```python
from build123d import *

# Parameters (mm, degrees)
SKETCH3_R           = 90
BOSS_EXTRUDE3_DEPTH = 2
SKETCH4_R           = 45
CUT_EXTRUDE1_DEPTH  = 2
BOSS_EXTRUDE4_DEPTH = 85
BOSS_EXTRUDE5_DEPTH = 85
CUT_EXTRUDE9_DEPTH  = 10
CIRPATTERN4_COUNT   = 3
CUT_EXTRUDE5_DEPTH  = 60
SKETCH15_W          = 5
SKETCH15_H          = 25
CUT_EXTRUDE10_DEPTH = 88.0000001
CIRPATTERN5_COUNT   = 3
SKETCH16_R          = 46
CUT_EXTRUDE11_DEPTH = 85
BOSS_EXTRUDE6_DEPTH = 2
SKETCH18_W          = 18.5
SKETCH18_H          = 12
CUT_EXTRUDE12_DEPTH = 2


with BuildPart() as part:
    # Sketch3 → Boss-Extrude3 (new body)
    with BuildSketch(Plane(origin=(0, 0, 0), x_dir=(1, 0, 0), z_dir=(0, 1, 0))):
        Circle(SKETCH3_R)
    extrude(amount=BOSS_EXTRUDE3_DEPTH)

    # Sketch4 → Cut-Extrude1 (cut)
    with BuildSketch(Plane.XZ):
        Circle(SKETCH4_R)
    extrude(amount=-CUT_EXTRUDE1_DEPTH, mode=Mode.SUBTRACT)

    # Sketch6 → Boss-Extrude4 (add)
    with BuildSketch(Plane.XZ):
        with BuildLine():
            Line((-46, 0), (-45, 0))
            ThreePointArc((-45, 0), (-41.574578963, 17.220754456), (-31.819805153, 31.819805153))
            Line((-31.819805153, 31.819805153), (-32.526911935, 32.526911935))
            ThreePointArc((-32.526911935, 32.526911935), (-42.498458496, 17.603437889), (-46, 0))
        make_face()
    boss_extrude4 = extrude(amount=BOSS_EXTRUDE4_DEPTH)

    # Sketch6<3> → Boss-Extrude5 (add)
    with BuildSketch(Plane.XZ):
        with BuildLine():
            Line((-50, 0), (-48, 0))
            ThreePointArc((-48, 0), (-44.346217561, 18.368804754), (-33.941125497, 33.941125497))
            Line((-33.941125497, 33.941125497), (-35.355339059, 35.355339059))
            ThreePointArc((-35.355339059, 35.355339059), (-46.193976626, 19.134171618), (-50, 0))
        make_face()
    boss_extrude5 = extrude(amount=BOSS_EXTRUDE5_DEPTH)

    # Sketch14 → Cut-Extrude9 (cut)
    with BuildSketch(Plane(origin=(-38.409902577, 0, 15.909902577), x_dir=(-0.382683432, 0, -0.923879533), z_dir=(0.923879533, 0, -0.382683432))):
        with BuildLine():
            Line((1.5, -75), (1.5, -83))
            ThreePointArc((1.5, -83), (0, -84.5), (-1.5, -83))
            Line((-1.5, -83), (-1.5, -75))
            ThreePointArc((-1.5, -75), (0, -73.5), (1.5, -75))
        make_face()
    cut_extrude9 = extrude(amount=-CUT_EXTRUDE9_DEPTH, mode=Mode.SUBTRACT)

    # CirPattern4: Boss-Extrude4, Boss-Extrude5, Cut-Extrude9 ×3 about axis
    cirpattern4_axis = Axis((0, 0, 0), (0, 1, 0))
    for i in range(1, CIRPATTERN4_COUNT):
        add(boss_extrude4.rotate(cirpattern4_axis, i * 360 / CIRPATTERN4_COUNT))
        add(boss_extrude5.rotate(cirpattern4_axis, i * 360 / CIRPATTERN4_COUNT))
        add(cut_extrude9.rotate(cirpattern4_axis, i * 360 / CIRPATTERN4_COUNT), mode=Mode.SUBTRACT)

    # Sketch11 → Cut-Extrude5 (cut, symmetric)
    with BuildSketch(Plane.XZ):
        Polygon((-6.747570404, -52.479477871), (11.40662685, -48.919264104), (13.715954699, -60.69495962), (-4.438242555, -64.255173387), align=None)
    extrude(amount=CUT_EXTRUDE5_DEPTH, both=True, mode=Mode.SUBTRACT)

    # Sketch15 → Cut-Extrude10 (cut, through all)
    with BuildSketch(Plane(origin=(0, 2, 0), x_dir=(1, 0, 0), z_dir=(0, 1, 0))):
        with Locations((57.5, -4.067185812)):
            Rectangle(SKETCH15_W, SKETCH15_H)
    cut_extrude10 = extrude(amount=-CUT_EXTRUDE10_DEPTH, mode=Mode.SUBTRACT)

    # CirPattern5: Cut-Extrude10 ×3 about axis
    cirpattern5_axis = Axis((0, 0, 0), (0, 1, 0))
    for i in range(1, CIRPATTERN5_COUNT):
        add(cut_extrude10.rotate(cirpattern5_axis, i * 360 / CIRPATTERN5_COUNT), mode=Mode.SUBTRACT)

    # Sketch16 → Cut-Extrude11 (cut)
    with BuildSketch(Plane.XZ.offset(85)):
        Circle(SKETCH16_R)
    extrude(amount=-CUT_EXTRUDE11_DEPTH, mode=Mode.SUBTRACT)

    # Sketch17 → Boss-Extrude6 (add)
    with BuildSketch(Plane(origin=(0, 2, 0), x_dir=(1, 0, 0), z_dir=(0, 1, 0))):
        Polygon((13.715954699, 60.69495962), (-4.438242555, 64.255173387), (-6.747570404, 52.479477871), (11.40662685, 48.919264104), align=None)
    extrude(amount=-BOSS_EXTRUDE6_DEPTH)

    # Sketch18 → Cut-Extrude12 (cut)
    with BuildSketch(Plane(origin=(0, 2, 0), x_dir=(1, 0, 0), z_dir=(0, 1, 0))):
        with Locations((9.25, -56)):
            Rectangle(SKETCH18_W, SKETCH18_H)
    extrude(amount=-CUT_EXTRUDE12_DEPTH, mode=Mode.SUBTRACT)


solid = part.part
```
The model under review builds one solid part; all positions refer to its coordinate system, in mm. A direction names the side the tool comes from. Coordinates: 2 decimals unless noted, no trailing zeros. Write each loop counter-clockwise with the first axis right and the second up, starting at its lowest first coordinate (ties: lowest second). Pieces come first, ordered by that corner, then holes.
1) We need section A-A on y = -6. State the section outline as (x, z) points.
2) We need section C-C on x = -2.5. State the section outline as (y, z) points, then the cut area to 3 significant figures.
3) Clearance check with flat-ended pins moving along their axes: pin 1 Ø8 at (x, z) = (-51, -25.5) entering from -Y; pin 2 Ø12 at (x, y) = (42, -63) entering from +Z; pin 3 Ø5 at (x, y) = (45.5, -12.5) entering from -Z. State where each tip first meets the part, or that it passes through.
4) Machinability: for faces 1 (the face through (6.3, -41.9, -49.6)), 2 (the face through (-31.174, 1.014, 45.51)), 3 (the face through (40, -42, 30)), 4 (the face through (-46.088, -41.905, 19.388)), which of the approach directions +Z, -Z, +X, -X, +Y, -Y give a long, thin tool a straight path to every point of the face, cutting with its end or side? Answer none if there is none.
5) To check wall thickness, follow probe 1 along X at (y, z) = (1, 0); probe 2 along Y at (x, z) = (-22, -44); probe 3 along X at (y, z) = (-78, 31.5). State the ranges of each line that lie inside material, in increasing order.
6) We need section D-D on z = -74. State the section outline as (x, y) points (3 decimals).
7) The part is to be moulded in two halves that separate along X. For faces 5 (the face through (38, -85, 30)), 6 (the face through (41.53, 0.986, 79.845)), 7 (the face through (20.765, 0.986, -39.923)), 8 (the face through (-44.45, -41.9, 18.12)), say which applies: pulls with the +X half, pulls with the -X half, needs draft (parallel to the pull), parting line crosses it, or undercut.
8) We need section B-B on z = -3. State the section outline as (x, y) points, then the cut area to 3 significant figures.
Answer list:
1. outline: (-50, 0) - (-48, 0) arc R48 cw to (-33.94, 33.94) - (-35.36, 35.36) arc R50 ccw to start; (-12.94, -48.3) arc R50 ccw to (25, -43.3) - (24, -41.57) arc R48 cw to (-12.42, -46.36) - close; (24, 41.57) arc R48 cw to (46.36, 12.42) - (48.3, 12.94) arc R50 ccw to (25, 43.3) - close
2. outline: (-85, -49.94) - (0, -49.94) - (0, -89.97) - (2, -89.97) - (2, -44.93) - (0, -44.93) - (0, -47.93) - (-85, -47.93) - close; (0, 44.93) - (2, 44.93) - (2, 89.97) - (0, 89.97) - close
2. area: 350 mm2
3. pin 1: stops at y = 0
3. pin 2: stops at z = 34.7
3. pin 3: stops at z = 12.42
4. face 1: -Z, -Y
4. face 2: +Y, -Y
4. face 3: +Z, +X, -Y
4. face 4: +Z, -X, -Y
5. probe 1: x = -90 to -45, 45 to 55, 60 to 90
5. probe 2: y = 0 to 2
5. probe 3: x = -38.83 to -36.22, 36.22 to 38.59
6. outline: (-51.225, 0) - (51.225, 0) - (51.225, 2) - (-51.225, 2) - close
7. face 5: needs draft
7. face 6: parting line crosses it
7. face 7: undercut
7. face 8: undercut
8. outline: (-89.95, 0) - (-44.9, 0) - (-44.9, 2) - (-89.95, 2) - close; (44.9, 0) - (55, 0) - (55, 2) - (44.9, 2) - close; (60, 0) - (89.95, 0) - (89.95, 2) - (60, 2) - close
8. area: 170 mm2
